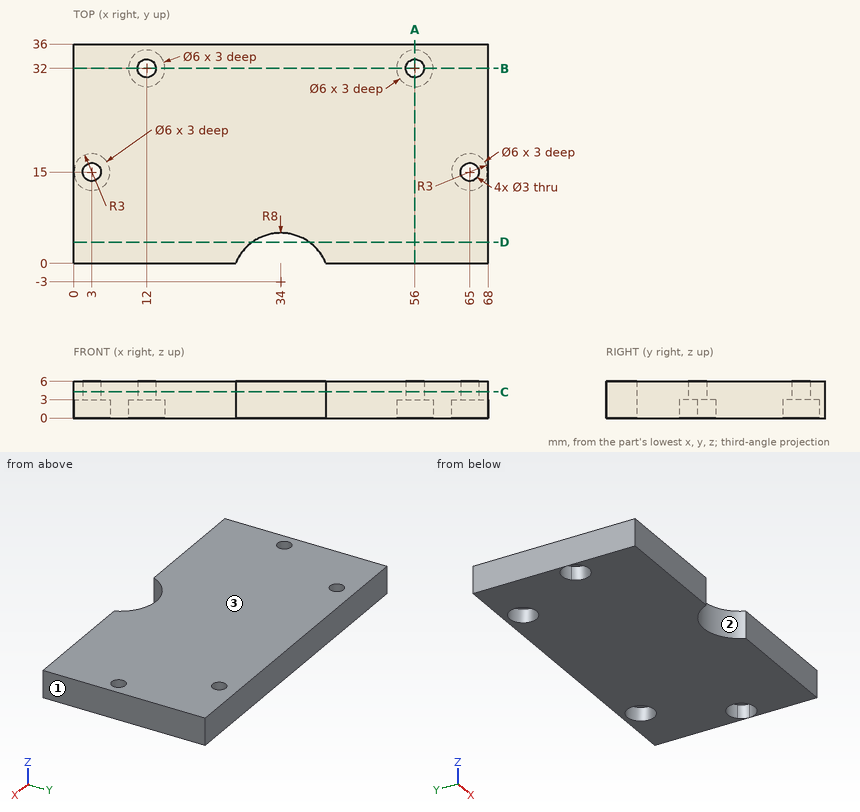
Verification items for this drawing (mm, ordinates from the low corner). Round coordinates to 2 decimals unless told otherwise and drop trailing zeros. Write each loop counter-clockwise with the first axis right and the second up, starting at its lowest first coordinate (ties: lowest second). Pieces come first, ordered by that corner, then holes. Notation, with made-up numbers: M 27,47.5 L 44,47.5 A33 ccw 44,83.5 Z; hole C 58,42.5 d3. An arc over 180 degrees is marked long. Write item = value, one per line. Start each with the question number.
1. Release check for a two-part mould opening along X. For the marked faces 1, 2 and 3 record: pulls with the +X half, pulls with the -X half, needs draft (parallel to the pull), parting line crosses it, or undercut.
2. Section check D-D, the plane y = 3.5. Record the cut outline in (x, z), then the cut area to 3 significant figures.
3. Scan lines: line 1 (X direction, y = 15, z = 5.05); line 2 (X direction, y = 32, z = 2.4); line 3 (Y direction, x = 3, z = 5.25). Record each from-to range of solid material in increasing order. Write a range as [from, to].
4. Section check A-A, the plane x = 56. Record the cut outline in (y, z), then the cut area to 3 significant figures.
5. Gauge pin test, flat end, axial feed: pin 1 (1.8 mm diameter, centred on x = 12.5, y = 33.5, fed in from -Z). Record the tip position at first contact, or that the pin passes through.
6. Section check C-C, the plane z = 4.3. Record the cut outline in (x, y).
7. Section check B-B, the plane y = 32. Record the cut outline in (x, z).
Results found:
q1.face_1 = pulls with the +X half
q1.face_2 = undercut
q1.face_3 = needs draft
q2.outline = M 0,0 L 29.34,0 L 29.34,6 L 0,6 Z; M 38.66,0 L 68,0 L 68,6 L 38.66,6 Z
q2.area = 352 mm^2
q3.line_1 = [0, 1.5], [4.5, 63.5], [66.5, 68]
q3.line_2 = [0, 9], [15, 53], [59, 68]
q3.line_3 = [0, 13.5], [16.5, 36]
q4.outline = M 0,0 L 29,0 L 29,3 L 30.5,3 L 30.5,6 L 0,6 Z; M 33.5,3 L 35,3 L 35,0 L 36,0 L 36,6 L 33.5,6 Z
q4.area = 189 mm^2
q5.pin_1 = 3
q6.outline = M 0,0 L 26.58,0 A8 cw 41.42,0 L 68,0 L 68,36 L 0,36 Z; hole C 3,15 d3; hole C 12,32 d3; hole C 56,32 d3; hole C 65,15 d3
q7.outline = M 0,0 L 9,0 L 9,3 L 10.5,3 L 10.5,6 L 0,6 Z; M 13.5,3 L 15,3 L 15,0 L 53,0 L 53,3 L 54.5,3 L 54.5,6 L 13.5,6 Z; M 57.5,3 L 59,3 L 59,0 L 68,0 L 68,6 L 57.5,6 Z
